Input: part model. Units: mm. Frame: model coordinates. Face numbers are marked on the shaded views. Give positions to 0.01 mm unless a question says otherwise; leave off trailing zeros. Loops run counter-clockwise (first coordinate to the right, second up) from the corner with the lowest first, then second, coordinate; pieces in that order, holes last. Notation, with made-up numbers: (-24.75, 0) - (-0.75, 0) arc R20 ccw to (-0.75, 37) - close; hole circle Ø11 at (-26.75, 26). An arc over 180 degrees is marked (long way). Answer as a JSON object with one key per item and string values.
Autodesk Inventor part; units mm, degrees
ref_plane "YZ Plane" through (0, 0, 0) normal (1, 0, 0) x (0, 1, 0)
ref_plane "XZ Plane" through (0, 0, 0) normal (0, 1, 0) x (-1, 0, 0)
ref_plane "XY Plane" through (0, 0, 0) normal (0, 0, 1) x (1, 0, 0)
sketch "Sketch1" plane through (0, 0, 0) normal (0, 1, 0) x (-1, 0, 0)
  line L0 (25, -25) -> (-25, -25)
  line L1 (-25, -25) -> (-25, 25)
  line L2 (-25, 25) -> (25, 25)
  line L3 (25, 25) -> (25, -25)
  line L4 (25, -25) -> (-25, 25) construction
  line L5 (-25, -25) -> (25, 25) construction
  point P0 (0, 0)
  dimension "d0" = 50
  dimension "d1" = 50
extrude "Extrusion1" add sketch "Sketch1" along normal blind 10
sketch "Sketch2" plane through (0, 10, 0) normal (0, 1, 0) x (1, 0, 0)
  circle A0 centre (0, 0) radius 7.55
  circle A1 centre (8.4853, 8.4853) radius 1.65
  line L0 (0, 0) -> (8.4853, 8.4853)
  line L1 (0, 0) -> (12, 0) construction
  circle A2 centre (-8.4853, 8.4853) radius 1.65
  circle A3 centre (-8.4853, -8.4853) radius 1.65
  circle A4 centre (8.4853, -8.4853) radius 1.65
  dimension "d4" = 15.1
  dimension "d5" = 3.3
  dimension "d7" = 12
  dimension "d8" = 45
  dimension "d11" = 360
extrude "lmk8uu holes" cut sketch "Sketch2" against normal up to next
equation "\"d4\" = center_hole"
equation "\"d5\" = mount_hole"
equation "\"d7\" = hole_radius"
equation "\"hole_radius\" = 12"
equation "\"mount_hole\" = 3.3"
equation "\"center_hole\" = 15.1"
properties part number "lmk8uugen"
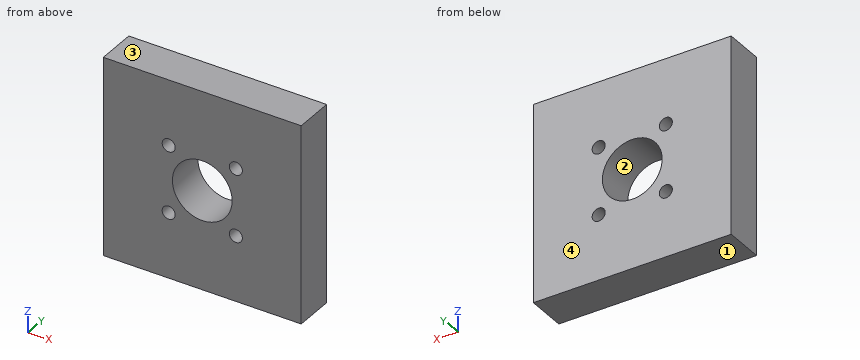
Item 1: Contact query for a flat-ended pin moving along its axis: P1, Ø3, axis at x = 8.49, z = 8.49, coming from the -Y side. Output: stop coordinate, or through.
Geometry check:
{"P1": "passes through"}
Item 2: Mould query, pull axis Z, two halves, no side actions, for the marked faces 1, 2, 3 and 4. Classes: released by +Z, released by -Z, zero draft, split by the parting line, or undercut.
Geometry check:
{"face 1": "released by -Z", "face 2": "undercut", "face 3": "released by +Z", "face 4": "zero draft"}
Item 3: Cut plane B-B (y = 6.25). Return loops of the section in (x, z).
Geometry check:
{"outline": "(-25, -25) - (25, -25) - (25, 25) - (-25, 25) - close; hole circle Ø3.3 at (-8.49, -8.49); hole circle Ø3.3 at (-8.49, 8.49); hole circle Ø15.1 at (0, 0); hole circle Ø3.3 at (8.49, -8.49); hole circle Ø3.3 at (8.49, 8.49)"}
Item 4: Material intervals for line 1 (Z direction, x = 0, y = 9.5); line 2 (X direction, y = 5.25, z = -9.5); line 3 (Z direction, x = -9, y = 1.5), sorted ascending. Write a range as [from, to].
Geometry check:
{"line 1": "z = [-25, -7.55], [7.55, 25]", "line 2": "x = [-25, -9.79], [-7.18, 7.18], [9.79, 25]", "line 3": "z = [-25, -10.05], [-6.92, 6.92], [10.05, 25]"}
Item 5: Cut plane A-A (x = 0). Return loops of the section in (y, z), then the cut area to 3 significant figures.
Geometry check:
{"outline": "(0, -25) - (10, -25) - (10, -7.55) - (0, -7.55) - close; (0, 7.55) - (10, 7.55) - (10, 25) - (0, 25) - close", "area": "349 mm2"}
